from build123d import *

# Parameters (mm, degrees)
BOSS_EXTRUDE2_DEPTH = 50


with BuildPart() as part:
    # Sketch1 → Boss-Extrude2 (new body)
    with BuildSketch(Plane(origin=(0, 0, 0), x_dir=(1, 0, 0), z_dir=(0, 1, 0))):
        with BuildLine():
            Line((5.999643171, -7.5), (7.5, -7.5))
            Line((7.5, -7.5), (7.5, 7.5))
            Line((7.5, 7.5), (-7.5, 7.5))
            Line((-7.5, 7.5), (-7.5, -7.5))
            Line((-7.5, -7.5), (-5.999643171, -7.5))
            Line((-5.999643171, -7.5), (-5.999643171, -11.193492834))
            ThreePointArc((-5.999643171, -11.193492834), (0, 12.7), (5.999643171, -11.193492834))
            Line((5.999643171, -11.193492834), (5.999643171, -7.5))
        make_face()
    extrude(amount=BOSS_EXTRUDE2_DEPTH)


solid = part.part
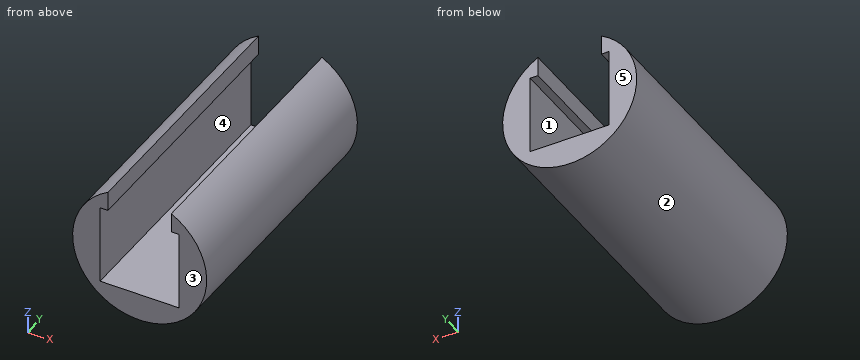
Here's how the part is built. I have some questions about the finished solid (model axes, mm). Face numbers are marked on the shaded views. A direction names the side the tool comes from. Give positions to 0.01 mm unless a question says otherwise; leave off trailing zeros. Order: outer loops, then holes, each group sorted by start corner. A loop starts at its lowest first (then second) coordinate and runs counter-clockwise, first axis right, second up. Notation, with made-up numbers: M 43.5,24 L 52.5,24 A24 ccw 52.5,52 Z; hole C 77.25,45.25 d11. An arc over 180 degrees is marked long. Answer as a JSON object with one key per item and string values. Group by question number.
1) I'm going to push flat-ended pins straight in: pin 1 Ø2 at (y, z) = (5, 4.5) entering from +X; pin 2 Ø5 at (x, y) = (-4.5, 27.5) entering from -Z; pin 3 Ø0.8 at (x, y) = (6.5, 34.5) entering from -Z. Where does each tip first touch, or does it pass through?
2) We'd pull the mould along Z, two halves only. Please class the marked faces 1, 2 and 3: pulls with the +Z half, pulls with the -Z half, needs draft (parallel to the pull), parting line crosses it, or undercut.
3) Suppose I cut it at A-A, the plane z = 0. Write out the boundary of the cut face in (x, y).
4) Suppose I cut it at C-C, the plane z = 4. Write out the boundary of the cut face in (x, y), plus the area to 3 significant figures.
5) Suppose I cut it at D-D, the plane x = 0. Write out the boundary of the cut face in (y, z), plus the area to 3 significant figures.
6) Suppose I cut it at B-B, the plane y = 33.5. Write out the boundary of the cut face in (x, z).
7) Please list where these lines run through material, in increasing order: L1, parallel to X at y = 34, z = 0; L2, parallel to X at y = 36, z = -7.25; L3, parallel to Z at x = -7, y = 41. Write a range as [from, to].
8) On a 3-axis mill with a long thin cutter (end or side, diameter ignored), from which of +Z, -Z, +X, -X, +Y, -Y can I reach the whole of each face in a straight line? I mean the marked faces 4 and 5. Say none if no direction works.
Results found:
{
 "1": {"pin 1": "x = 12.21", "pin 2": "z = -12.54", "pin 3": "z = -11.14"},
 "2": {"face 1": "undercut", "face 2": "parting line crosses it", "face 3": "needs draft"},
 "3": {"outline": "M -12.7,0 L -7.5,0 L -7.5,50 L -12.7,50 Z; M 7.5,0 L 12.7,0 L 12.7,50 L 7.5,50 Z"},
 "4": {"outline": "M -12.05,0 L -7.5,0 L -7.5,50 L -12.05,50 Z; M 7.5,0 L 12.05,0 L 12.05,50 L 7.5,50 Z", "area": "455 mm²"},
 "5": {"outline": "M 0,-12.7 L 50,-12.7 L 50,-7.5 L 0,-7.5 Z", "area": "260 mm²"},
 "6": {"outline": "M -7.5,-7.5 L -7.5,7.5 L -6,7.5 L -6,11.19 A12.7 ccw long 6,11.19 L 6,7.5 L 7.5,7.5 L 7.5,-7.5 Z"},
 "7": {"L1": "[-12.7, -7.5], [7.5, 12.7]", "L2": "[-10.43, -7.5], [7.5, 10.43]", "L3": "[-10.6, -7.5], [7.5, 10.6]"},
 "8": {"face 4": "+Y, -Y", "face 5": "+Z, -Z, +X, -X, +Y"}
}
